Here's the drawing with two shaded views (mm, measured from the low corner). I have some questions. A direction names the side the tool comes from. Give positions to 0.01 mm unless a question says otherwise; leave off trailing zeros. Write each loop counter-clockwise with the first axis right and the second up, starting at its lowest first coordinate (ties: lowest second). Pieces come first, ordered by that corner, then holes.
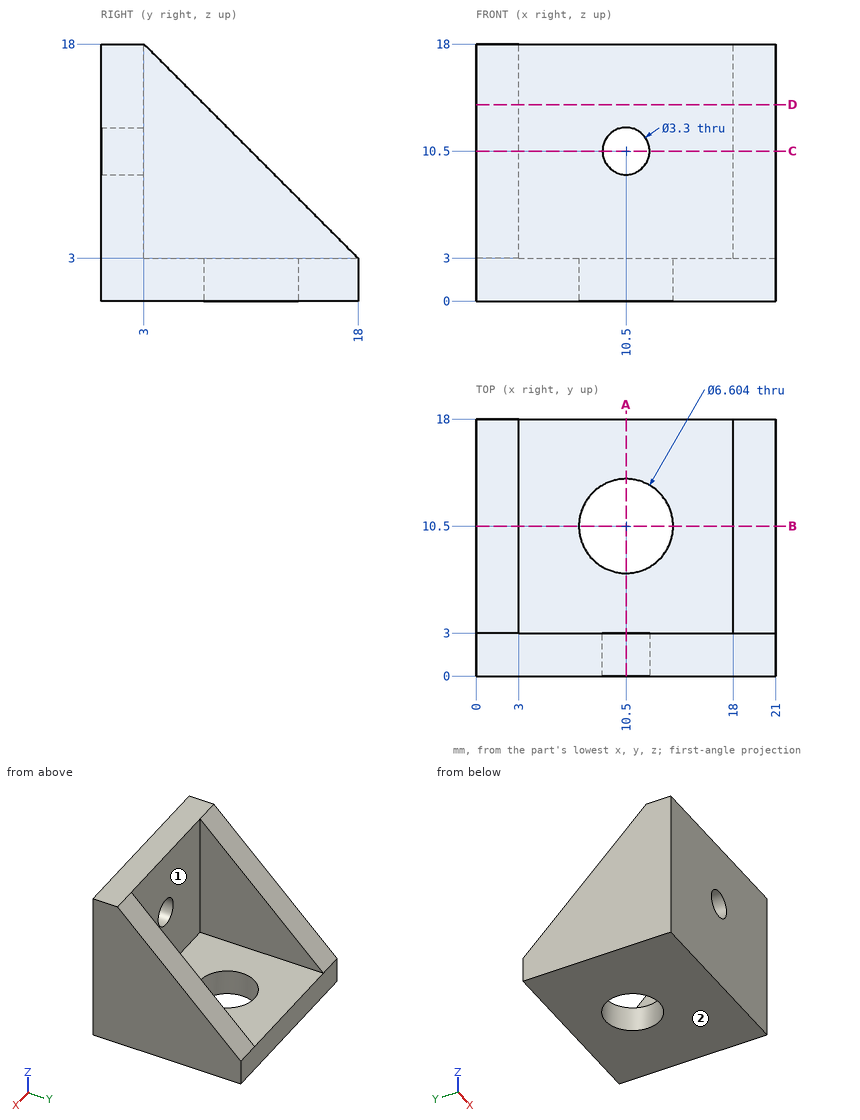
(1) For the marked faces 1 and 2, which set-ups out of +Z, -Z, +X, -X, +Y, -Y let a thin tool reach every point of the face, with its end or its side?
Returned:
face 1: +Z, +Y
face 2: -Z, +X, -X, +Y, -Y
(2) If I drill on L1, parallel to X at y = 5.25, z = 13.5; L2, parallel to Y at x = 10.5, z = 1.2; L3, parallel to Z at x = 17.5, y = 12.5, over which ranges is the centre line in solid material (lowest first)?
Returned:
L1: x = 0 to 3, 18 to 21
L2: y = 0 to 7.2, 13.8 to 18
L3: z = 0 to 3
(3) Imagine slicing it at A-A, the plane x = 10.5. Write out the boundary of the cut face in (y, z), plus the area to 3 significant figures.
Returned:
outline: (0, 0) - (7.2, 0) - (7.2, 3) - (3, 3) - (3, 8.85) - (0, 8.85) - close; (0, 12.15) - (3, 12.15) - (3, 18) - (0, 18) - close; (13.8, 0) - (18, 0) - (18, 3) - (13.8, 3) - close
area: 69.3 mm2
(4) Will these pins go through, and if not, where does the flat tip stop? P1, Ø5, axis at y = 3, z = 9.5, coming from the -X side; P2, Ø8.5, axis at x = 10.5, y = 10.5, coming from the +Z side; P3, Ø4.5, axis at x = 11.5, z = 13.5, coming from the +Y side.
Returned:
P1: stops at x = 0
P2: stops at z = 3
P3: stops at y = 3
(5) Imagine slicing it at C-C, the plane z = 10.5. Write out the boundary of the cut face in (x, y), plus the area to 3 significant figures.
Returned:
outline: (0, 0) - (8.85, 0) - (8.85, 3) - (3, 3) - (3, 10.5) - (0, 10.5) - close; (12.15, 0) - (21, 0) - (21, 10.5) - (18, 10.5) - (18, 3) - (12.15, 3) - close
area: 98.1 mm2
(6) Imagine slicing it at B-B, the plane y = 10.5. Write out the boundary of the cut face in (x, z), plus the area to 3 significant figures.
Returned:
outline: (0, 0) - (7.2, 0) - (7.2, 3) - (3, 3) - (3, 10.5) - (0, 10.5) - close; (13.8, 0) - (21, 0) - (21, 10.5) - (18, 10.5) - (18, 3) - (13.8, 3) - close
area: 88.2 mm2
(7) Imagine slicing it at D-D, the plane z = 13.75. Write out the boundary of the cut face in (x, y), plus the area to 3 significant figures.
Returned:
outline: (0, 0) - (21, 0) - (21, 7.25) - (18, 7.25) - (18, 3) - (3, 3) - (3, 7.25) - (0, 7.25) - close
area: 88.5 mm2
